```python
from build123d import *

# Parameters (mm, degrees)
SKETCH1_W           = 84
SKETCH1_H           = 84
BOSS_EXTRUDE1_DEPTH = 22
SKETCH2_W           = 80
SKETCH2_H           = 80
CUT_EXTRUDE1_DEPTH  = 42
SKETCH3_W           = 6
SKETCH3_H           = 8
CUT_EXTRUDE2_DEPTH  = 73.746133918
CUT_EXTRUDE3_REACH  = 98.457
SKETCH5_W           = 79
SKETCH5_H           = 20
BOSS_EXTRUDE2_DEPTH = 10
CUT_EXTRUDE4_REACH  = 98.457
SKETCH6_R           = 13
SKETCH8_W           = 2
SKETCH8_H           = 42
BOSS_EXTRUDE3_DEPTH = 14
CUT_EXTRUDE6_REACH  = 100.914
SKETCH7_R           = 1
SKETCH7_W           = 9
SKETCH7_H           = 9
SKETCH9_R           = 1.5
CUT_EXTRUDE7_DEPTH  = 82.633326528
SKETCH14_R          = 14.5
BOSS_EXTRUDE4_DEPTH = 13
SKETCH15_R          = 12.5
CUT_EXTRUDE8_DEPTH  = 11
CUT_EXTRUDE9_REACH  = 102.578
SKETCH16_R          = 3


with BuildPart() as part:
    # Sketch1 → Boss-Extrude1 (new, symmetric)
    with BuildSketch(Plane(origin=(0, 0, 0), x_dir=(1, 0, 0), z_dir=(0, 1, 0))):
        Rectangle(SKETCH1_W, SKETCH1_H)
    extrude(amount=BOSS_EXTRUDE1_DEPTH, both=True)

    # Sketch2 → Cut-Extrude1 (cut)
    with BuildSketch(Plane(origin=(0, 22, 0), x_dir=(1, 0, 0), z_dir=(0, 1, 0))):
        Rectangle(SKETCH2_W, SKETCH2_H)
    extrude(amount=-CUT_EXTRUDE1_DEPTH, mode=Mode.SUBTRACT)

    # Sketch3 → Cut-Extrude2 (cut, through all)
    with BuildSketch(Plane(origin=(0, -20, 0), x_dir=(1, 0, 0), z_dir=(0, 1, 0))):
        with Locations((33, 27.1)):
            Rectangle(SKETCH3_W, SKETCH3_H)
    extrude(amount=-CUT_EXTRUDE2_DEPTH, mode=Mode.SUBTRACT)

    # Sketch5 → Cut-Extrude3 (cut, up to next)
    with BuildSketch(Plane(origin=(42, 0, 0), x_dir=(0, 0, -1), z_dir=(1, 0, 0)), mode=Mode.PRIVATE) as cut_extrude3_sk1:
        with Locations((0, -10)):
            Rectangle(SKETCH5_W, SKETCH5_H)
    cut_extrude3_tool1 = extrude(cut_extrude3_sk1.sketch, amount=-CUT_EXTRUDE3_REACH, mode=Mode.PRIVATE) & part.part
    add(cut_extrude3_tool1.solids().sort_by_distance((42, -10, 0))[0], mode=Mode.SUBTRACT)

    # Sketch4 → Boss-Extrude2 (add)
    with BuildSketch(Plane(origin=(-40, 0, 0), x_dir=(0, 0, -1), z_dir=(1, 0, 0))):
        Polygon((-22, 4), (-20, 4), (-20, 2), (20, 2), (20, 4), (22, 4), (24, 4), (24, 2), (22, 2), (22, 0), (-22, 0), align=None)
    boss_extrude2 = extrude(amount=BOSS_EXTRUDE2_DEPTH)

    # Mirror1: Boss-Extrude2 across plane
    add(boss_extrude2.mirror(Plane(origin=(0, 0, 0), x_dir=(0, 0, 1), z_dir=(1, 0, 0))))

    # Sketch6 → Cut-Extrude4 (cut, up to next)
    with BuildSketch(Plane(origin=(0, 0, -42), x_dir=(-1, 0, 0), z_dir=(0, 0, -1)), mode=Mode.PRIVATE) as cut_extrude4_sk1:
        with Locations((-19.5, 17)):
            Circle(SKETCH6_R)
    cut_extrude4_tool1 = extrude(cut_extrude4_sk1.sketch, amount=-CUT_EXTRUDE4_REACH, mode=Mode.PRIVATE) & part.part
    add(cut_extrude4_tool1.solids().sort_by_distance((19.5, 17, -42))[0], mode=Mode.SUBTRACT)

    # Sketch8 → Boss-Extrude3 (add)
    with BuildSketch(Plane(origin=(0, 22, 0), x_dir=(1, 0, 0), z_dir=(0, 1, 0))):
        with Locations((-41, 21)):
            Rectangle(SKETCH8_W, SKETCH8_H)
    extrude(amount=BOSS_EXTRUDE3_DEPTH)

    # Sketch7 → Cut-Extrude6 (cut, up to next)
    with BuildSketch(Plane(origin=(-40, 0, 0), x_dir=(0, 0, -1), z_dir=(1, 0, 0)), mode=Mode.PRIVATE) as cut_extrude6_sk1:
        with Locations((31, 32)):
            Circle(SKETCH7_R)
    cut_extrude6_tool1 = extrude(cut_extrude6_sk1.sketch, amount=-CUT_EXTRUDE6_REACH, mode=Mode.PRIVATE) & part.part
    # Sketch7 → Cut-Extrude6 (cut, up to next)
    with BuildSketch(Plane(origin=(-40, 0, 0), x_dir=(0, 0, -1), z_dir=(1, 0, 0)), mode=Mode.PRIVATE) as cut_extrude6_sk2:
        with Locations((31, 20)):
            Circle(SKETCH7_R)
    cut_extrude6_tool2 = extrude(cut_extrude6_sk2.sketch, amount=-CUT_EXTRUDE6_REACH, mode=Mode.PRIVATE) & part.part
    # Sketch7 → Cut-Extrude6 (cut, up to next)
    with BuildSketch(Plane(origin=(-40, 0, 0), x_dir=(0, 0, -1), z_dir=(1, 0, 0)), mode=Mode.PRIVATE) as cut_extrude6_sk3:
        with Locations((11, 20)):
            Circle(SKETCH7_R)
    cut_extrude6_tool3 = extrude(cut_extrude6_sk3.sketch, amount=-CUT_EXTRUDE6_REACH, mode=Mode.PRIVATE) & part.part
    # Sketch7 → Cut-Extrude6 (cut, up to next)
    with BuildSketch(Plane(origin=(-40, 0, 0), x_dir=(0, 0, -1), z_dir=(1, 0, 0)), mode=Mode.PRIVATE) as cut_extrude6_sk4:
        with Locations((11, 32)):
            Circle(SKETCH7_R)
    cut_extrude6_tool4 = extrude(cut_extrude6_sk4.sketch, amount=-CUT_EXTRUDE6_REACH, mode=Mode.PRIVATE) & part.part
    # Sketch7 → Cut-Extrude6 (cut, up to next)
    with BuildSketch(Plane(origin=(-40, 0, 0), x_dir=(0, 0, -1), z_dir=(1, 0, 0)), mode=Mode.PRIVATE) as cut_extrude6_sk5:
        with Locations((21, 20)):
            Rectangle(SKETCH7_W, SKETCH7_H)
    cut_extrude6_tool5 = extrude(cut_extrude6_sk5.sketch, amount=-CUT_EXTRUDE6_REACH, mode=Mode.PRIVATE) & part.part
    add(cut_extrude6_tool1.solids().sort_by_distance((-40, 32, -31))[0], mode=Mode.SUBTRACT)
    add(cut_extrude6_tool2.solids().sort_by_distance((-40, 20, -31))[0], mode=Mode.SUBTRACT)
    add(cut_extrude6_tool3.solids().sort_by_distance((-40, 20, -11))[0], mode=Mode.SUBTRACT)
    add(cut_extrude6_tool4.solids().sort_by_distance((-40, 32, -11))[0], mode=Mode.SUBTRACT)
    add(cut_extrude6_tool5.solids().sort_by_distance((-40, 20, -21))[0], mode=Mode.SUBTRACT)

    # Sketch9 → Cut-Extrude7 (cut, through all)
    with BuildSketch(Plane(origin=(0, -20, 0), x_dir=(1, 0, 0), z_dir=(0, 1, 0))):
        with Locations(Location((-25, 25, 0), (0, 0, 270))):
            Circle(SKETCH9_R)
        with Locations(Location((25, 25, 0), (0, 0, 270))):
            Circle(SKETCH9_R)
        with Locations(Location((25, -25, 0), (0, 0, 270))):
            Circle(SKETCH9_R)
        with Locations(Location((-25, -25, 0), (0, 0, 270))):
            Circle(SKETCH9_R)
    extrude(amount=-CUT_EXTRUDE7_DEPTH, mode=Mode.SUBTRACT)

    # Sketch14 → Boss-Extrude4 (add)
    with BuildSketch(Plane.XY.offset(-40)):
        with Locations((-15, -5)):
            Circle(SKETCH14_R)
    boss_extrude4 = extrude(amount=-BOSS_EXTRUDE4_DEPTH)

    # Sketch15 → Cut-Extrude8 (cut)
    with BuildSketch(Plane(origin=(0, 0, -53), x_dir=(-1, 0, 0), z_dir=(0, 0, -1))):
        with Locations((15, -5)):
            Circle(SKETCH15_R)
    cut_extrude8 = extrude(amount=-CUT_EXTRUDE8_DEPTH, mode=Mode.SUBTRACT)

    # Sketch16 → Cut-Extrude9 (cut, up to next)
    with BuildSketch(Plane(origin=(0, 0, -42), x_dir=(-1, 0, 0), z_dir=(0, 0, -1)), mode=Mode.PRIVATE) as cut_extrude9_sk1:
        with Locations((15, -5)):
            Circle(SKETCH16_R)
    cut_extrude9_tool1 = extrude(cut_extrude9_sk1.sketch, amount=-CUT_EXTRUDE9_REACH, mode=Mode.PRIVATE) & part.part
    cut_extrude9 = cut_extrude9_tool1.solids().sort_by_distance((-15, -5, -42))[0]
    add(cut_extrude9, mode=Mode.SUBTRACT)

    # Mirror2: Boss-Extrude4, Cut-Extrude8, Cut-Extrude9 across plane
    add(boss_extrude4.mirror(Plane.XY))
    add(cut_extrude8.mirror(Plane.XY), mode=Mode.SUBTRACT)
    add(cut_extrude9.mirror(Plane.XY), mode=Mode.SUBTRACT)


solid = part.part
```
Can you work these out from the model? Positions are in its coordinate system, mm. A direction names the side the tool comes from. Coordinates: 2 decimals unless noted, no trailing zeros. Loops run counter-clockwise (first coordinate to the right, second up) from the corner with the lowest first, then second, coordinate; pieces in that order, holes last.
1) Which directions (+Z, -Z, +X, -X, +Y, -Y) give clear straight access to the entire face, cutting with the end or side of a thin tool? Please do faces 1 (the flat face through (-35, 0, 0)), 2 (the flat face through (-18, -8, -42)), 3 (the cylindrical face through (-12.79, -2.97, 41.01)), 4 (the flat face through (-35, 2, 0)), 5 (the cylindrical face through (-5.08, -12.606, 47.577)).
2) Thinking about a two-plate mould opening in Y: for faces 6 (the cylindrical face through (-23.99, -20.99, -26.11)), 7 (the flat face through (-40, 8, 0)), 8 (the flat face through (35, 4, -22)), which applies, pulls with the +Y half, pulls with the -Y half, needs draft (parallel to the pull), parting line crosses it, or undercut?
3) Imagine slicing it at A-A on x = -33.5. List the corners of the cut face in (y, z) for me, plus the area to 3 significant figures.
4) Imagine slicing it at C-C on z = -6.5. List the corners of the cut face in (x, y) for me.
5) Imagine slicing it at D-D on y = 17. List the corners of the cut face in (x, z) for me.
6) I need wall thicknesses on probe 1 along Y at (x, z) = (-37, -3); probe 2 along Z at (x, y) = (21.5, -2). Which ranges of each line are inside material? Lowest first, please.
7) Imagine slicing it at B-B on x = -15. State how many separate pieces and enclosed holes the cut face has, plus the area to 3 significant figures.
8) For pin 1 (1 mm diameter, centred on x = -40.5, y = 19, fed in from -Z); pin 2 (1 mm diameter, centred on y = -6.5, z = -35, fed in from +X); pin 3 (2 mm diameter, centred on x = 32.5, y = -21, fed in from +Z), each with a flat end and sliding along its axis, tell me the tip position at first contact or that it passes through.
Completed:
1. face 1: +X
1. face 2: -Z
1. face 3: +Z, -Z
1. face 4: +Y
1. face 5: +Z
2. face 6: needs draft
2. face 7: undercut
2. face 8: pulls with the +Y half
3. outline: (-22, -42) - (22, -42) - (22, -40) - (-20, -40) - (-20, 40) - (22, 40) - (22, 42) - (-22, 42) - close; (0, -22) - (2, -22) - (2, -24) - (4, -24) - (4, -20) - (2, -20) - (2, 20) - (4, 20) - (4, 22) - (0, 22) - close
3. area: 436 mm2
4. outline: (-42, -22) - (42, -22) - (42, -20) - (-40, -20) - (-40, 0) - (-30, 0) - (-30, 2) - (-40, 2) - (-40, 36) - (-42, 36) - close; (30, 0) - (42, 0) - (42, 22) - (40, 22) - (40, 2) - (30, 2) - close
5. outline: (-42, -42) - (6.5, -42) - (6.5, -40) - (-40, -40) - (-40, -25.5) - (-42, -25.5) - close; (-42, -16.5) - (-40, -16.5) - (-40, 40) - (40, 40) - (40, -40) - (32.5, -40) - (32.5, -42) - (42, -42) - (42, 42) - (-42, 42) - close
6. probe 1: y = -22 to -20, 0 to 2
6. probe 2: z = -42 to -40, 40 to 42
7. separate pieces: 3
7. enclosed holes: 0
7. area: 400 mm2
8. pin 1: stops at z = -42
8. pin 2: stops at x = -40
8. pin 3: stops at z = 42
